Design review of the part built by this model. Coordinates are the model's own, in mm. Coordinates: 2 decimals unless noted, no trailing zeros. Loops run counter-clockwise (first coordinate to the right, second up) from the corner with the lowest first, then second, coordinate; pieces in that order, holes last. Notation, with made-up numbers: (80, 87.25) -> (124, 87.25) arc R32 cw to (124, 119.25) -> close; hole circle Ø9 at (82.25, 2.5). An arc over 180 degrees is marked (long way). Use CSV: the item, a comma, the result in double quotes.
```python
from build123d import *

# Parameters (mm, degrees)
SKETCH1_W                                         = 20.5
SKETCH1_H                                         = 20.5
SKETCH1_R                                         = 6.25
BOSS_EXTRUDE1_DEPTH                               = 20
SKETCH2_W                                         = 20.5
SKETCH2_H                                         = 20
BOSS_EXTRUDE2_DEPTH                               = 10
LPATTERN1_COUNT                                   = 4
LPATTERN1_PITCH                                   = 30
SKETCH3_W                                         = 9.5
SKETCH3_H                                         = 30.5
BOSS_EXTRUDE3_DEPTH                               = 20
CSK_FOR_8_FLAT_HEAD_MACHINE_SCREW_100_D           = 4.9149
CSK_FOR_8_FLAT_HEAD_MACHINE_SCREW_100_CSINK_D     = 8.4328
CSK_FOR_8_FLAT_HEAD_MACHINE_SCREW_100_CSINK_ANGLE = 100
FILLET1_R                                         = 8
CHAMFER1_SIZE                                     = 1


with BuildPart() as part:
    # Sketch1 → Boss-Extrude1 (new body)
    with BuildSketch(Plane(origin=(0, 0, 0), x_dir=(1, 0, 0), z_dir=(0, 1, 0))):
        Rectangle(SKETCH1_W, SKETCH1_H)
        Circle(SKETCH1_R, mode=Mode.SUBTRACT)
    extrude(amount=BOSS_EXTRUDE1_DEPTH)

    # Sketch2 → Boss-Extrude2 (add)
    with BuildSketch(Plane(origin=(0, 0, -10.25), x_dir=(-1, 0, 0), z_dir=(0, 0, -1))):
        with Locations((0, 10)):
            Rectangle(SKETCH2_W, SKETCH2_H)
    extrude(amount=BOSS_EXTRUDE2_DEPTH)


with BuildPart() as lpattern1_1:
    # LPattern1: pattern copy
    add(part.part.moved(Location(Vector(1, 0, 0) * (1 * LPATTERN1_PITCH))))


with BuildPart() as lpattern1_2:
    # LPattern1: pattern copy
    add(part.part.moved(Location(Vector(1, 0, 0) * (2 * LPATTERN1_PITCH))))


with BuildPart() as lpattern1_3:
    # LPattern1: pattern copy
    add(part.part.moved(Location(Vector(1, 0, 0) * (3 * LPATTERN1_PITCH))))


with BuildPart() as part_1:
    add(part.part)

    add(lpattern1_1.part)  # Boss-Extrude3 merges LPattern1_1

    add(lpattern1_2.part)  # Boss-Extrude3 merges LPattern1_2

    add(lpattern1_3.part)  # Boss-Extrude3 merges LPattern1_3
    # Sketch3 → Boss-Extrude3 (add)
    with BuildSketch(Plane(origin=(0, 20, 0), x_dir=(1, 0, 0), z_dir=(0, 1, 0))):
        with Locations((15, 5)):
            Rectangle(SKETCH3_W, SKETCH3_H)
        with Locations((45, 5)):
            Rectangle(SKETCH3_W, SKETCH3_H)
        with Locations((75, 5)):
            Rectangle(SKETCH3_W, SKETCH3_H)
    extrude(amount=-BOSS_EXTRUDE3_DEPTH)

    # CSK for #8 Flat Head Machine Screw (100)1 (through all)
    with Locations(Plane(origin=(15, 10, 10.25), x_dir=(1, 0, 0), z_dir=(0, 0, 1))):
        with Locations((0, 0), (30, 0), (60, 0)):
            CounterSinkHole(CSK_FOR_8_FLAT_HEAD_MACHINE_SCREW_100_D / 2, CSK_FOR_8_FLAT_HEAD_MACHINE_SCREW_100_CSINK_D / 2, counter_sink_angle=CSK_FOR_8_FLAT_HEAD_MACHINE_SCREW_100_CSINK_ANGLE)

    # Fillet1
    fillet1_edges = [part_1.edges().sort_by_distance(p)[0] for p in [
        (-10.25, 10, -20.25),
        (-10.25, 10, 10.25),
        (100.25, 10, 10.25),
        (100.25, 10, -20.25),
    ]]
    fillet(fillet1_edges, radius=FILLET1_R)

    # Chamfer1
    chamfer1_edges = [part_1.edges().sort_by_distance(p)[0] for p in [
        (45, 20, -20.25),
        (45, 0, -20.25),
        (45, 20, 10.25),
        (100.25, 20, -5),
        (-10.25, 20, -5),
        (-7.906854249, 20, 7.906854249),
        (97.906854249, 20, 7.906854249),
        (97.906854249, 20, -17.906854249),
        (-7.906854249, 20, -17.906854249),
        (-10.25, 0, -5),
        (-6.25, 0, 0),
        (100.25, 0, -5),
        (45, 0, 10.25),
        (-7.906854249, 0, 7.906854249),
        (-6.25, 20, 0),
        (97.906854249, 0, 7.906854249),
        (97.906854249, 0, -17.906854249),
        (-7.906854249, 0, -17.906854249),
        (23.75, 0, 0),
        (23.75, 20, 0),
        (53.75, 0, 0),
        (53.75, 20, 0),
        (83.75, 0, 0),
        (83.75, 20, 0),
    ]]
    chamfer(chamfer1_edges, length=CHAMFER1_SIZE)


solid = part_1.part
```
Item 1: To check wall thickness, follow line 1 along X through (y, z) = (14.75, 0); line 2 along Y through (x, z) = (75, -1.5); line 3 along Z through (x, y) = (30, 15.75). State the ranges of each line that lie inside material, in increasing order.
Checked values:
line 1,"-10.25 to -6.25, 6.25 to 23.75, 36.25 to 53.75, 66.25 to 83.75, 96.25 to 100.25"
line 2,"0 to 7.54, 12.46 to 20"
line 3,"-20.25 to -6.25, 6.25 to 10.25"
Item 2: Add section A-A (y = 10). State how many separate pieces and enclosed holes the cut face has, then the cut area to 3 significant figures.
Checked values:
separate pieces,"4"
enclosed holes,"4"
area,"2,370 mm^2"
Item 3: Clearance check with flat-ended pins moving along their axes: pin 1 (8 mm diameter, centred on x = 15, y = 10, fed in from +Z); pin 2 (5.5 mm diameter, centred on x = 45, y = 10, fed in from +Z). State where each tip first meets the part, or that it passes through.
Checked values:
pin 1,"z = 10.07"
pin 2,"z = 9.02"
Item 4: Draft analysis for pull direction Y (two halves, no side actions). For faces 1 (the face through (44, 20, -5)), 2 (the face through (72.73, 9.06, -5.94)), 3 (the face through (-7.844, 10.126, -17.969)), state which applies: pulls with the +Y half, pulls with the -Y half, needs draft (parallel to the pull), parting line crosses it, or undercut.
Checked values:
face 1,"pulls with the +Y half"
face 2,"undercut"
face 3,"needs draft"
Item 5: Add section C-C (y = 17). Give the boundary of the cut face in (x, z), then the cut area to 3 significant figures.
Checked values:
outline,"(-10.25, -12.25) arc R8 ccw to (-2.25, -20.25) -> (92.25, -20.25) arc R8 ccw to (100.25, -12.25) -> (100.25, 2.25) arc R8 ccw to (92.25, 10.25) -> (-2.25, 10.25) arc R8 ccw to (-10.25, 2.25) -> close; hole circle Ø12.5 at (0, 0); hole circle Ø12.5 at (30, 0); hole circle Ø12.5 at (60, 0); hole circle Ø12.5 at (90, 0)"
area,"2,820 mm^2"
Item 6: Add section B-B (x = 0). Give the boundary of the cut face in (y, z).
Checked values:
outline,"(0, -19.25) -> (1, -20.25) -> (19, -20.25) -> (20, -19.25) -> (20, -7.25) -> (19, -6.25) -> (1, -6.25) -> (0, -7.25) -> close; (0, 7.25) -> (1, 6.25) -> (19, 6.25) -> (20, 7.25) -> (20, 9.25) -> (19, 10.25) -> (1, 10.25) -> (0, 9.25) -> close"
